Autodesk Inventor part; units mm, degrees
ref_plane "YZ Plane" through (0, 0, 0) normal (1, 0, 0) x (0, 1, 0)
ref_plane "XZ Plane" through (0, 0, 0) normal (0, 1, 0) x (-1, 0, 0)
ref_plane "XY Plane" through (0, 0, 0) normal (0, 0, 1) x (1, 0, 0)
sketch "Sketch1" plane through (0, 0, 0) normal (1, 0, 0) x (0, 1, 0)
  line L0 (6.0871, 13.8808) -> (-19.3129, 13.8808)
  line L1 (-19.3129, 13.8808) -> (-19.3129, -316.3192)
  line L2 (-19.3129, -316.3192) -> (6.0871, -316.3192)
  line L3 (6.0871, -316.3192) -> (6.0871, 13.8808)
  circle A0 centre (-12.9629, -11.5192) radius 2.3368
  circle A1 centre (-12.9629, -290.9192) radius 2.3368
  line L4 (-19.3129, -151.2192) -> (65.5988, -151.2192) construction
  circle A2 centre (94.9871, -125.8192) radius 2.3368
  circle A3 centre (94.9871, -176.6192) radius 2.3368
  line L5 (94.9871, -125.8192) -> (94.9871, -176.6192) construction
  line L6 (-12.9629, -11.5192) -> (-12.9629, -290.9192) construction
  line L7 (102.6071, -119.4692) -> (102.6071, -182.9692)
  line L8 (6.0871, -11.5192) -> (15.6121, -11.5192) construction
  line L9 (6.0871, -290.9192) -> (15.6121, -290.9192) construction
  line L10 (6.0871, 13.8808) -> (15.6121, -11.5192)
  line L11 (6.0871, -316.3192) -> (15.6121, -290.9192)
  line L12 (102.6071, -119.4692) -> (15.6121, -11.5192)
  line L13 (102.6071, -182.9692) -> (15.6121, -290.9192)
  line L14 (102.6071, -119.4692) -> (134.3571, -119.4692)
  line L15 (134.3571, -119.4692) -> (134.3571, -182.9692)
  line L16 (134.3571, -182.9692) -> (102.6071, -182.9692)
  line L17 (102.6071, -182.9692) -> (102.6071, -119.4692)
  line L18 (102.6071, -182.9692) -> (117.44, -194.9228)
  line L19 (15.6121, -290.9192) -> (30.445, -302.8728)
  line L20 (117.44, -194.9228) -> (30.445, -302.8728)
  line L21 (102.6071, -119.4692) -> (117.44, -107.5156)
  line L22 (117.44, -107.5156) -> (30.445, 0.4344)
  line L23 (30.445, 0.4344) -> (15.6121, -11.5192)
  point P0 (0, 0)
  dimension "d0" = 25.4
  dimension "d1" = 330.2
  dimension "d2" = 4.6736
  dimension "d3" = 4.6736
  dimension "d4" = 279.4
  dimension "d5" = 25.4
  dimension "d6" = 6.35
  dimension "d7" = 84.9117
  dimension "d8" = 4.6736
  dimension "d9" = 4.6736
  dimension "d10" = 50.8
  dimension "d11" = 25.4
  dimension "d12" = 107.95
  dimension "d13" = 7.62
  dimension "d14" = 9.525
  dimension "d15" = 9.525
  dimension "d16" = 63.5
  dimension "d17" = 6.35
  dimension "d18" = 31.75
  dimension "d19" = 19.05
  dimension "d20" = 19.05
ref_plane "Work Plane1" through (1.5875, 0, 0) normal (1, 0, 0) x (0, 0, -1)
extrude "Plate1" add sketch "Sketch1" along normal blind 3.048
sketch "Sketch3" plane through (0, 0, 0) normal (-1, 0, 0) x (0, 0, 1)
  circle A0 centre (-176.6192, 94.9871) radius 2.3368
  circle A1 centre (-125.8192, 94.9871) radius 2.3368
  circle A2 centre (-11.5192, -12.9629) radius 2.3368
  circle A3 centre (-290.9192, -12.9629) radius 2.3368
  line L0 (-107.5156, 117.44) -> (0.4344, 30.445)
  line L1 (-119.4692, 102.6071) -> (-107.5156, 117.44)
  line L2 (-119.4692, 134.3571) -> (-119.4692, 102.6071)
  line L3 (-182.9692, 134.3571) -> (-119.4692, 134.3571)
  line L4 (-182.9692, 102.6071) -> (-182.9692, 134.3571)
  line L5 (-194.9228, 117.44) -> (-182.9692, 102.6071)
  line L6 (-302.8728, 30.445) -> (-194.9228, 117.44)
  line L7 (-290.9192, 15.6121) -> (-302.8728, 30.445)
  line L8 (-316.3192, 6.0871) -> (-290.9192, 15.6121)
  line L9 (-316.3192, -19.3129) -> (-316.3192, 6.0871)
  line L10 (13.8808, -19.3129) -> (-316.3192, -19.3129)
  line L11 (13.8808, 6.0871) -> (13.8808, -19.3129)
  line L12 (-11.5192, 15.6121) -> (13.8808, 6.0871)
  line L13 (0.4344, 30.445) -> (-11.5192, 15.6121)
  line L14 (-151.2192, 134.3571) -> (-151.2192, -19.3129)
  point P0 (0, 0)
extrude "Cut1" cut sketch "Sketch3" against normal blind 3.048 contours L0 L13 L12 L11 L10 L14 L3 L2 L1
equation "\"d24\" = Thickness"
equation "\"d23\" = Thickness"
equation "\"BendRadius\" = Thickness"
equation "\"BendReliefWidth\" = Thickness"
equation "\"BendReliefDepth\" = 0.5 * Thickness"
equation "\"CornerReliefSize\" = 4 * Thickness"
equation "\"MinimumRemnant\" = 2 * Thickness"
equation "\"TransitionRadius\" = BendRadius"
equation "\"JacobiRadiusSize\" = BendRadius"
equation "\"GapSize\" = Thickness"
properties part number "backpanel"
Verification items for the finished model (mm, model axes). A direction names the side the tool comes from. Give positions to 0.01 mm unless a question says otherwise; leave off trailing zeros. Order: outer loops, then holes, each group sorted by start corner. A loop starts at its lowest first (then second) coordinate and runs counter-clockwise, first axis right, second up. Notation, with made-up numbers: (-15, -30.5) -> (-3, -30.5) arc R20 cw to (-3, -23.5) -> close; hole circle Ø9 at (-24, -30.5). An arc over 180 degrees is marked (long way). Answer as CSV lines item,"result".
Q1. Access from +Z, -Z, +X, -X, +Y, -Y to the whole of each face (thin tool, end or side, straight path). Record for faces 1 (the flat face through (1.5, 22.92, -296.81)), 2 (the cylindrical face through (1.5, 94.48, -174.34)), 3 (the flat face through (1.5, 109.92, -188.86)).
Solutions:
face 1,"-Z, +X, -X"
face 2,"+X, -X"
face 3,"+X, -X, +Y"
Q2. Scan lines: probe 1 along Y at (x, z) = (2.2, -295.5); probe 2 along Y at (x, z) = (2.15, -297); probe 3 along Z at (x, y) = (0.1, 123.5). Record each from-to range of solid material in increasing order.
Solutions:
probe 1,"y = -19.31 to 13.89, 21.3 to 36.39"
probe 2,"y = -19.31 to 13.33, 23.16 to 35.18"
probe 3,"z = -182.97 to -151.22"
Q3. Release check for a two-part mould opening along Y. For faces 4 (the flat face through (1.503, 74.551, -248.142)), 5 (the flat face through (3.048, 39, -214)), 6 (the cylindrical face through (1.503, -13.267, -293.236)) record: +Y half, -Y half, draft (parallel to the pull), parting line (faces both ways), or undercut.
Solutions:
face 4,"+Y half"
face 5,"draft"
face 6,"undercut"
Q4. Sectioned sample at B-B on x = 0.8. Record the cut outline in (y, z) (3 decimals), plus the area to 3 significant figures.
Solutions:
outline,"(-19.313, -316.319) -> (6.087, -316.319) -> (15.612, -290.919) -> (30.445, -302.873) -> (117.44, -194.923) -> (102.607, -182.969) -> (134.357, -182.969) -> (134.357, -151.219) -> (-19.313, -151.219) -> close; hole circle Ø4.674 at (-12.963, -290.919); hole circle Ø4.674 at (94.987, -176.619)"
area,"16,700 mm²"
Q5. Sectioned sample at D-D on y = 11. Record the cut outline in (x, z), plus the area to 3 significant figures.
Solutions:
outline,"(0, -303.22) -> (3.05, -303.22) -> (3.05, -151.22) -> (0, -151.22) -> close"
area,"463 mm²"
Q6. Sectioned sample at A-A on y = 112. Record the cut outline in (x, z).
Solutions:
outline,"(0, -201.67) -> (3.05, -201.67) -> (3.05, -190.54) -> (0, -190.54) -> close; (0, -182.97) -> (3.05, -182.97) -> (3.05, -151.22) -> (0, -151.22) -> close"
Q7. Sectioned sample at C-C on z = -197.5. Record the cut outline in (x, y).
Solutions:
outline,"(0, -19.31) -> (3.05, -19.31) -> (3.05, 115.36) -> (0, 115.36) -> close"
Q8. Depth check by flat-ended pin: pin 1 (6 mm diameter, centred on y = -12.96, z = -290.92, fed in from -X); pin 2 (3 mm diameter, centred on y = 94.99, z = -176.62, fed in from +X). Enter the tip coordinate at first touch or a pass-through.
Solutions:
pin 1,"stops at x = 0"
pin 2,"passes through"
